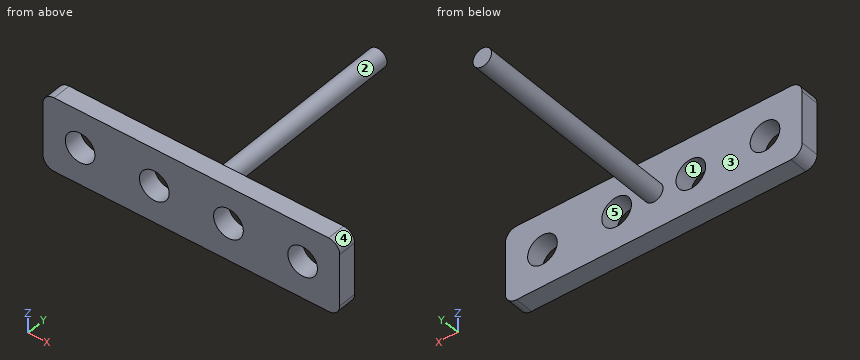
```python
from build123d import *

# Parameters (mm, degrees)
SKETCH1_W             = 80
SKETCH1_H             = 20
BOSS_EXTRUDE1_DEPTH   = 2.5
F_8_0MM_DOWEL_HOLE1_D = 8
SKETCH6_R             = 2.5
BOSS_EXTRUDE2_DEPTH   = 60
FILLET1_R             = 3


with BuildPart() as part:
    # Sketch1 → Boss-Extrude1 (new, symmetric)
    with BuildSketch(Plane(origin=(0, 0, 0), x_dir=(1, 0, 0), z_dir=(0, 1, 0))):
        Rectangle(SKETCH1_W, SKETCH1_H)
    extrude(amount=BOSS_EXTRUDE1_DEPTH, both=True)

    # Ø8.0mm Dowel Hole1 (through all)
    with Locations(Plane(origin=(0, 2.5, 0), x_dir=(1, 0, 0), z_dir=(0, 1, 0))):
        with Locations((-30, 0), (-10, 0), (10, 0), (30, 0)):
            Hole(F_8_0MM_DOWEL_HOLE1_D / 2)

    # Sketch6 → Boss-Extrude2 (add)
    with BuildSketch(Plane(origin=(0, 0, 0), x_dir=(1, 0, 0), z_dir=(0, 1, 0))):
        with Locations(Location((0, 0, 0), (0, 0, 90))):
            Circle(SKETCH6_R)
    extrude(amount=BOSS_EXTRUDE2_DEPTH)

    # Fillet1
    fillet1_edges = [part.edges().sort_by_distance(p)[0] for p in [
        (40, 0, 10),
        (-40, 0, 10),
        (-40, 0, -10),
        (40, 0, -10),
    ]]
    fillet(fillet1_edges, radius=FILLET1_R)


solid = part.part
```
CAD build for the part. Positions are in the model's coordinates, mm. Face numbers are marked on the shaded views. A direction names the side the tool comes from. Coordinates: 2 decimals unless noted, no trailing zeros. Order: outer loops, then holes, each group sorted by start corner. A loop starts at its lowest first (then second) coordinate and runs counter-clockwise, first axis right, second up. Notation, with made-up numbers: M 1,76.25 L 48,76.25 A24 cw 48,102.25 Z; hole C 53.5,52 d4. An arc over 180 degrees is marked long. Answer as CSV lines item,"result".
1) Cut at A-A (z = 0). List the corners of the cut face in (x, y).
Verdict:
outline,"M -40,-2.5 L -34,-2.5 L -34,2.5 L -40,2.5 Z; M -26,-2.5 L -14,-2.5 L -14,2.5 L -26,2.5 Z; M -6,-2.5 L 6,-2.5 L 6,2.5 L 2.5,2.5 L 2.5,60 L -2.5,60 L -2.5,2.5 L -6,2.5 Z; M 14,-2.5 L 26,-2.5 L 26,2.5 L 14,2.5 Z; M 34,-2.5 L 40,-2.5 L 40,2.5 L 34,2.5 Z"
2) Flat gauge pins, fed straight in: P1, Ø8, axis at x = -20, z = -5.5, coming from the +Y side; P2, Ø4, axis at x = -10.5, y = 4, coming from the +Z side; P3, Ø4, axis at y = 51.5, z = -4, coming from the +X side. Where does each tip first touch, or does it go through?
Verdict:
P1,"y = 2.5"
P2,"z = 10"
P3,"x = 1.5"
3) Drill centre lines: L1, parallel to Z at x = -10, y = 0.2; L2, parallel to Y at x = -13.5, z = 4.75; L3, parallel to X at y = 15, z = -0.25. Where is each one in solid material? Low to high. Write a range as from..to.
Verdict:
L1,"-10..-4, 4..10"
L2,"-2.5..2.5"
L3,"-2.49..2.49"
4) Cut at D-D (y = 6.5). List the corners of the cut face in (x, z), then the cut area to 3 significant figures.
Verdict:
outline,"C 0,0 d5"
area,"19.6 mm2"
5) 3-axis set-ups, long thin cutter, end or side, ignore diameter. For the marked faces 1 and 2: which of +Z, -Z, +X, -X, +Y, -Y reach the whole face in a straight line?
Verdict:
face 1,"+Y, -Y"
face 2,"+Y"
6) Cut at B-B (x = 10). List the corners of the cut face in (y, z).
Verdict:
outline,"M -2.5,-10 L 2.5,-10 L 2.5,-4 L -2.5,-4 Z; M -2.5,4 L 2.5,4 L 2.5,10 L -2.5,10 Z"
7) Mould opens along Z. For the marked faces 3, 4 and 5 say: released by +Z, released by -Z, zero draft, split by the parting line, or undercut.
Verdict:
face 3,"zero draft"
face 4,"released by +Z"
face 5,"undercut"
8) Cut at C-C (x = 0). List the corners of the cut face in (y, z).
Verdict:
outline,"M -2.5,-10 L 2.5,-10 L 2.5,-2.5 L 60,-2.5 L 60,2.5 L 2.5,2.5 L 2.5,10 L -2.5,10 Z"
